Part model, mm, in its own coordinate system. Give positions to 0.01 mm unless a question says otherwise; leave off trailing zeros. Order: outer loops, then holes, each group sorted by start corner. A loop starts at its lowest first (then second) coordinate and runs counter-clockwise, first axis right, second up.
Autodesk Inventor part; units mm, degrees
ref_plane "YZ Plane" through (0, 0, 0) normal (1, 0, 0) x (0, 1, 0)
ref_plane "XZ Plane" through (0, 0, 0) normal (0, 1, 0) x (-1, 0, 0)
ref_plane "XY Plane" through (0, 0, 0) normal (0, 0, 1) x (1, 0, 0)
sketch "Sketch1" plane through (0, 0, 0) normal (0, 1, 0) x (-1, 0, 0)
  line L0 (0, 0) -> (25.4, 0)
  line L1 (25.4, 0) -> (25.4, -50.8)
  line L2 (25.4, -50.8) -> (0, -50.8)
  line L3 (0, -50.8) -> (0, 0)
  line L4 (3.175, -3.175) -> (22.225, -3.175)
  line L5 (22.225, -3.175) -> (22.225, -47.625)
  line L6 (22.225, -47.625) -> (3.175, -47.625)
  line L7 (3.175, -47.625) -> (3.175, -3.175)
  dimension "d0" = 50.8
  dimension "d1" = 25.4
  dimension "d2" = 3.175
extrude "Extrusion1" add sketch "Sketch1" along normal blind 889
sketch "Sketch6" plane through (0, 0, 0) normal (1, 0, 0) x (0, 0, -1)
  circle A0 centre (25.4, 768.35) radius 12.7
  line L0 (0, 889) -> (50.8, 889)
  line L1 (0, 0) -> (0, 889)
  dimension "d5" = 25.4
  dimension "d6" = 120.65
  dimension "d7" = 25.4
extrude "Extrusion2" cut sketch "Sketch6" against normal blind 25.4
sketch "Sketch8" plane through (-25.4, 0, 0) normal (0, 0, 1) x (1, 0, 0)
  circle A0 centre (12.7, 31.75) radius 2.0701
  line L0 (0, 0) -> (0, 889)
  line L1 (25.4, 0) -> (0, 0)
  dimension "d13" = 4.1402
  dimension "d14" = 12.7
  dimension "d15" = 31.75
extrude "Extrusion3" cut sketch "Sketch8" against normal blind 76.2
sketch "Sketch9" plane through (-25.4, 0, 0) normal (0, 0, 1) x (1, 0, 0)
  circle A0 centre (12.7, 157.5054) radius 2.0701
  line L0 (25.4, 0) -> (0, 0)
  line L1 (0, 0) -> (0, 889)
  dimension "d18" = 4.1402
  dimension "d19" = 157.5054
  dimension "d20" = 12.7
extrude "Extrusion4" cut sketch "Sketch9" against normal blind 76.2
sketch "Sketch10" plane through (0, 0, 0) normal (1, 0, 0) x (0, 0, -1)
  circle A0 centre (25.4, 528.066) radius 12.7
  line L0 (50.8, 0) -> (50.8, 889)
  line L1 (50.8, 0) -> (0, 0)
  circle A1 centre (25.4, 666.75) radius 12.7
  dimension "d23" = 25.4
  dimension "d24" = 25.4
  dimension "d25" = 528.066
  dimension "d26" = 25.4
  dimension "d27" = 666.75
extrude "Extrusion5" cut sketch "Sketch10" against normal blind 25.4
properties part number "16in 2x1 Aluminum Block-ver1-1111-2019"
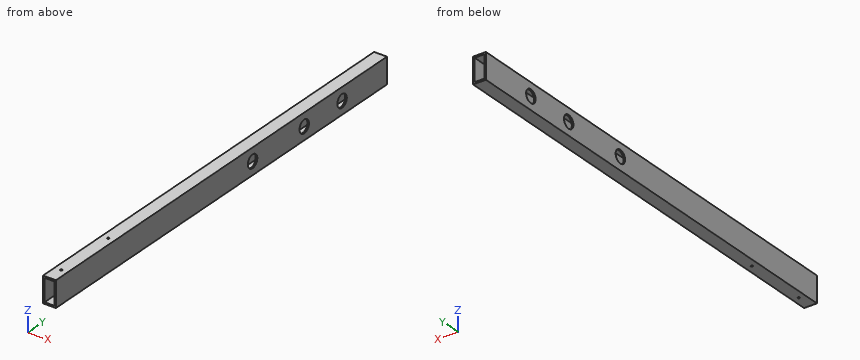
Item 1: Drill centre lines: probe 1 along Y at (x, z) = (-1.7, -25.4); probe 2 along Y at (x, z) = (-12.7, -49.65); probe 3 along X at (y, z) = (278, -41) (3 decimals). Where is each one in solid material? Low to high.
Item 2: Band-saw the part on B-B on z = -25.4. Give the number of separate pieces and of enclosed holes in the cut face, plus the area to 3 significant figures.
Item 3: Band-saw the part on A-A on y = 666.75. List the corners of the cut face in (x, z) (3 decimals), plus the area to 3 significant figures.
Item 4: Drop flat-ended pins along their axis: P1, Ø20.5, axis at y = 528.066, z = -25.4, coming from the +X side; P2, Ø5, axis at x = -12.7, y = 157.51, coming from the -Z side. Give the stop position or say it passes through.
Working result:
1. probe 1: y = 0 to 515.37, 540.77 to 654.05, 679.45 to 755.65, 781.05 to 889
1. probe 2: y = 0 to 29.68, 33.82 to 155.44, 159.58 to 889
1. probe 3: x = -25.4 to -22.225, -3.175 to 0
2. separate pieces: 8
2. enclosed holes: 0
2. area: 5,160 mm2
3. outline: (-25.4, -50.8) - (0, -50.8) - (0, -38.1) - (-3.175, -38.1) - (-3.175, -47.625) - (-22.225, -47.625) - (-22.225, -38.1) - (-25.4, -38.1) - close; (-25.4, -12.7) - (-22.225, -12.7) - (-22.225, -3.175) - (-3.175, -3.175) - (-3.175, -12.7) - (0, -12.7) - (0, 0) - (-25.4, 0) - close
3. area: 282 mm2
4. P1: passes through
4. P2: stops at z = -50.8
